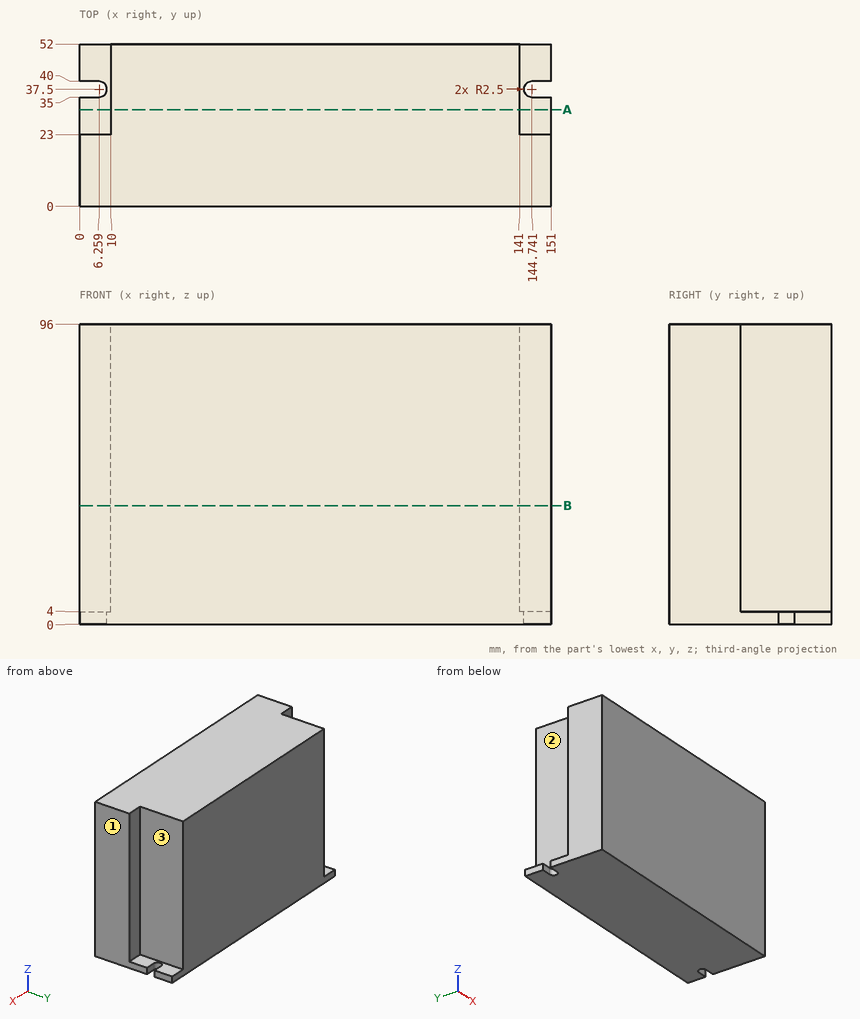
Input: dimensioned drawing with shaded views. Units: mm. Origin: part minimum x, y, z. A direction names the side the tool comes from. Coordinates: 2 decimals unless noted, no trailing zeros. Order: outer loops, then holes, each group sorted by start corner. A loop starts at its lowest first (then second) coordinate and runs counter-clockwise, first axis right, second up. Notation, with made-up numbers: M 14,-16.75 L 21,-16.75 A20 ccw 21,6.25 Z; hole C 53,-29 d1. An arc over 180 degrees is marked long. Answer as CSV lines item,"result".
Q1. Line query: probe 1 along X at (y, z) = (24, 27.5). Output: solid intervals per line, ascending. Write a range as [from, to].
Answers:
probe 1,"x = [10, 141]"
Q2. Section A-A on y = 31. Return the cut outline in (x, z), and give its area (3 significant figures).
Answers:
outline,"M 0,0 L 151,0 L 151,4 L 141,4 L 141,96 L 10,96 L 10,4 L 0,4 Z"
area,"12,700 mm^2"
Q3. First-contact query: P1, Ø3, axis at y = 35, z = 85.5, coming from the -X side; P2, Ø5, axis at x = 146.5, z = 62.5, coming from the +Y side; P3, Ø23, axis at y = 41.5, z = 70.5, coming from the +X side. Flat tips, straight axial feed; report the tip coordinate or a pass-through.
Answers:
P1,"stops at x = 10"
P2,"stops at y = 23"
P3,"stops at x = 141"
Q4. Set-up query: the marked faces 1, 2 and 3. Return all of +Z, -Z, +X, -X, +Y, -Y with unobstructed straight access to the full face (end or side cutting, diameter ignored); none if empty.
Answers:
face 1,"+Z, -Z, +X, +Y, -Y"
face 2,"+Z, -X, +Y"
face 3,"+Z, +X, +Y"
Q5. Section B-B on z = 38. Return the cut outline in (x, y).
Answers:
outline,"M 0,0 L 151,0 L 151,23 L 141,23 L 141,52 L 10,52 L 10,23 L 0,23 Z"
